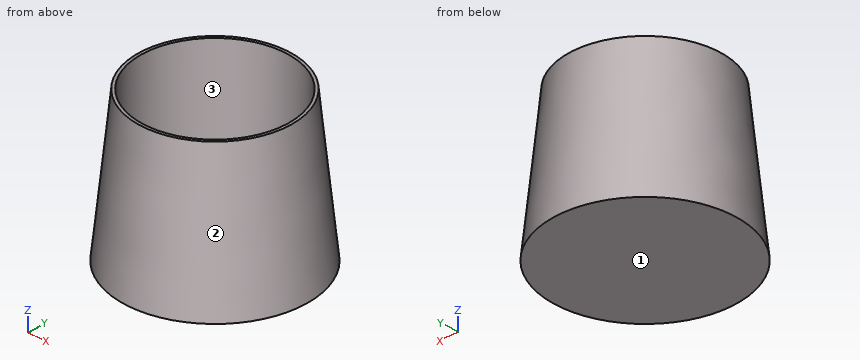
```python
from build123d import *

# Parameters (mm, degrees)
F0_R     = 63.5
F0_R_2   = 50.8
F1_DEPTH = 101.6
F2_DEPTH = 12.7
F3_SIZE2 = 10.67858
F3_SIZE  = 101.59999


# Not quite as in the source:
# - a fillet or chamfer is up to 0.001 mm smaller than in the source, because OpenCascade refuses the exact size


with BuildPart() as f1:
    # F0 (on Top) → F1 (new body)
    with BuildSketch(Plane.XY):
        Circle(F0_R)
        Circle(F0_R_2, mode=Mode.SUBTRACT)
    extrude(amount=F1_DEPTH)

    # F0 (on Top) → F2 (join)
    with BuildSketch(Plane.XY):
        Circle(F0_R_2)
    extrude(amount=F2_DEPTH)

    # F3 (size 101.6 and 10.678590303 in the source; OpenCascade refuses exactly that, so slightly less here)
    f3_edges = [f1.edges().sort_by_distance(p)[0] for p in [
        (-63.5, 0, 101.6),
    ]]
    f3_side = f1.faces().sort_by_distance((-63.5, 0, 50.8))[0]
    chamfer(f3_edges, length=F3_SIZE, length2=F3_SIZE2, reference=f3_side)


solid = f1.part
```
Model file for the job. Use its own axes, mm. Face numbers are marked on the shaded views. Coordinates: 2 decimals unless noted, no trailing zeros. Write each loop counter-clockwise with the first axis right and the second up, starting at its lowest first coordinate (ties: lowest second). Pieces come first, ordered by that corner, then holes. Notation, with made-up numbers: (82.5, 38) - (132.5, 38) arc R26 cw to (132.5, 73) - close; hole circle Ø9 at (25.5, 8). An arc over 180 degrees is marked (long way). Use a Markdown table: item, result. Add a question column.
Item 1: Band-saw the part on D-D, the plane z = 34. Write the cut outline in (x, y), and give its area (3 significant figures).
Item 2: Band-saw the part on C-C, the plane z = 82.5. Write the cut outline in (x, y).
Item 3: Drill centre lines: line 1 along Z through (x, y) = (44, -18); line 2 along X through (y, z) = (31.5, 34.5); line 3 along Y through (x, z) = (-25, 23). Where is each one in solid material? Low to high.
Item 4: Drop flat-ended pins along their axis: pin 1 (3 mm diameter, centred on x = -47.5, z = 84, fed in from +Y); pin 2 (1 mm diameter, centred on x = -44, y = -16.5, fed in from +Z); pin 3 (2 mm diameter, centred on y = -23, z = 91.5, fed in from -X); pin 4 (12 mm diameter, centred on x = 7, y = -14, fed in from -Z). Give the stop position or say it passes through.
Item 5: Two-plate mould, pull along X, no slides. Class the marked faces 1, 2 and 3: pulls with the +X half, pulls with the -X half, needs draft (parallel to the pull), parting line crosses it, or undercut.
A:
| question | item | result |
|---|---|---|
| 1 | outline | circle Ø119.85 at (0, 0); hole circle Ø101.6 at (0, 0) |
| 1 | area | 3,170 mm² |
| 2 | outline | circle Ø109.66 at (0, 0); hole circle Ø101.6 at (0, 0) |
| 3 | line 1 | z = 0 to 12.7 |
| 3 | line 2 | x = -50.92 to -39.85, 39.85 to 50.92 |
| 3 | line 3 | y = -55.73 to -44.22, 44.22 to 55.73 |
| 4 | pin 1 | stops at y = 29.56 |
| 4 | pin 2 | stops at z = 12.7 |
| 4 | pin 3 | stops at x = -49.2 |
| 4 | pin 4 | stops at z = 0 |
| 5 | face 1 | needs draft |
| 5 | face 2 | parting line crosses it |
| 5 | face 3 | undercut |
